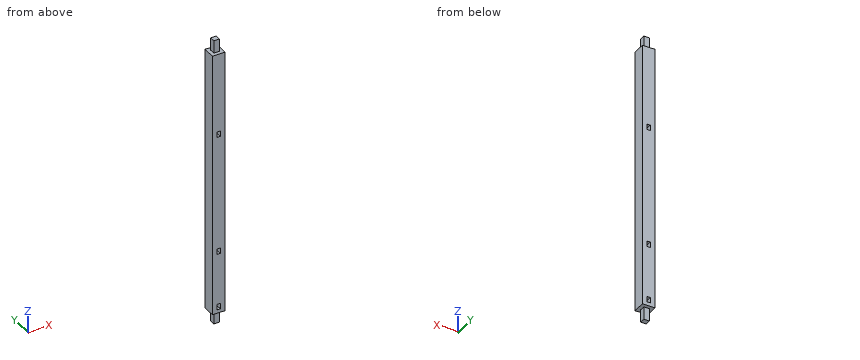
```python
from build123d import *

# Parameters (mm, degrees)
F0_W     = 101.6
F0_H     = 101.6
F1_DEPTH = 1168.4
F2_W     = 101.6
F2_H     = 101.6
F2_W_2   = 44.45
F2_H_2   = 44.45
F3_DEPTH = 101.6
F4_W     = 25.4
F4_H     = 44.45
F5_DEPTH = 101.601
F6_W     = 25.4
F6_H     = 44.45
F7_DEPTH = 101.601
F8_W     = 25.4
F8_H     = 44.45
F9_DEPTH = 101.601


# Not quite as in the source:
# - a pattern or mirror of a feature is missing from the dataset's text; its kind, count and spacing are read off the source's solid


with BuildPart() as f1:
    # F0 (on Top) → F1 (new body, symmetric)
    with BuildSketch(Plane.XY):
        Rectangle(F0_W, F0_H)
    extrude(amount=F1_DEPTH, both=True)

    # F2 (on face) → F3 (cut)
    with BuildSketch(Plane.XY.offset(1168.4)):
        Rectangle(F2_W, F2_H)
        Rectangle(F2_W_2, F2_H_2, mode=Mode.SUBTRACT)
    f3 = extrude(amount=-F3_DEPTH, mode=Mode.SUBTRACT)

    # F3_copies: F3 across plane
    add(f3.mirror(Plane(origin=(0, 0, 0), x_dir=(-1, 0, 0), z_dir=(0, 0, -1))), mode=Mode.SUBTRACT)

    # F4 (on face) → F5 (cut, through all)
    with BuildSketch(Plane.XZ.offset(50.8)):
        with Locations((0, 406.4)):
            Rectangle(F4_W, F4_H)
    extrude(amount=-F5_DEPTH, mode=Mode.SUBTRACT)

    # F6 (on face) → F7 (cut, through all)
    with BuildSketch(Plane(origin=(0, 50.8, 0), x_dir=(-1, 0, 0), z_dir=(0, 1, 0))):
        with Locations((0, -558.8)):
            Rectangle(F6_W, F6_H)
    extrude(amount=-F7_DEPTH, mode=Mode.SUBTRACT)

    # F8 (on face) → F9 (cut, through all)
    with BuildSketch(Plane(origin=(0, 50.8, 0), x_dir=(-1, 0, 0), z_dir=(0, 1, 0))):
        with Locations((0, -1016)):
            Rectangle(F8_W, F8_H)
    extrude(amount=-F9_DEPTH, mode=Mode.SUBTRACT)


solid = f1.part
```
Here's how the part is built. I have some questions about the finished solid (model axes, mm). Round coordinates to 2 decimals unless told otherwise and drop trailing zeros. Write each loop counter-clockwise with the first axis right and the second up, starting at its lowest first coordinate (ties: lowest second). Pieces come first, ordered by that corner, then holes.
Q1. Please list where these lines run through material, in increasing order: probe 1 along Z at (x, y) = (9, 12.5) (3 decimals); probe 2 along Z at (x, y) = (10.5, 35.5) (3 decimals); probe 3 along Z at (x, y) = (43, -44.5).
Q2. Will these pins go through, and if not, where does the flat tip stop? P1, Ø13.5, axis at x = 4.5, z = 1093.5, coming from the -Y side (3 decimals); P2, Ø10, axis at x = -33.5, y = 1, coming from the +Z side; P3, Ø13.5, axis at y = -3, z = -1099, coming from the +X side (3 decimals).
Q3. If we section it at A-A on y = -6: Write out the boundary of the cut face in (x, z) (3 decimals), plus the area to 3 significant figures.
Answer below:
1. probe 1: z = -1168.4 to -1038.225, -993.775 to -581.025, -536.575 to 384.175, 428.625 to 1168.4
1. probe 2: z = -1066.8 to -1038.225, -993.775 to -581.025, -536.575 to 384.175, 428.625 to 1066.8
1. probe 3: z = -1066.8 to 1066.8
2. P1: stops at y = -22.225
2. P2: stops at z = 1066.8
2. P3: stops at x = 22.225
3. outline: (-50.8, -1066.8) - (-22.225, -1066.8) - (-22.225, -1168.4) - (22.225, -1168.4) - (22.225, -1066.8) - (50.8, -1066.8) - (50.8, 1066.8) - (22.225, 1066.8) - (22.225, 1168.4) - (-22.225, 1168.4) - (-22.225, 1066.8) - (-50.8, 1066.8) - close; hole (-12.7, -1038.225) - (12.7, -1038.225) - (12.7, -993.775) - (-12.7, -993.775) - close; hole (-12.7, -581.025) - (12.7, -581.025) - (12.7, -536.575) - (-12.7, -536.575) - close; hole (-12.7, 384.175) - (12.7, 384.175) - (12.7, 428.625) - (-12.7, 428.625) - close
3. area: 222,000 mm2
